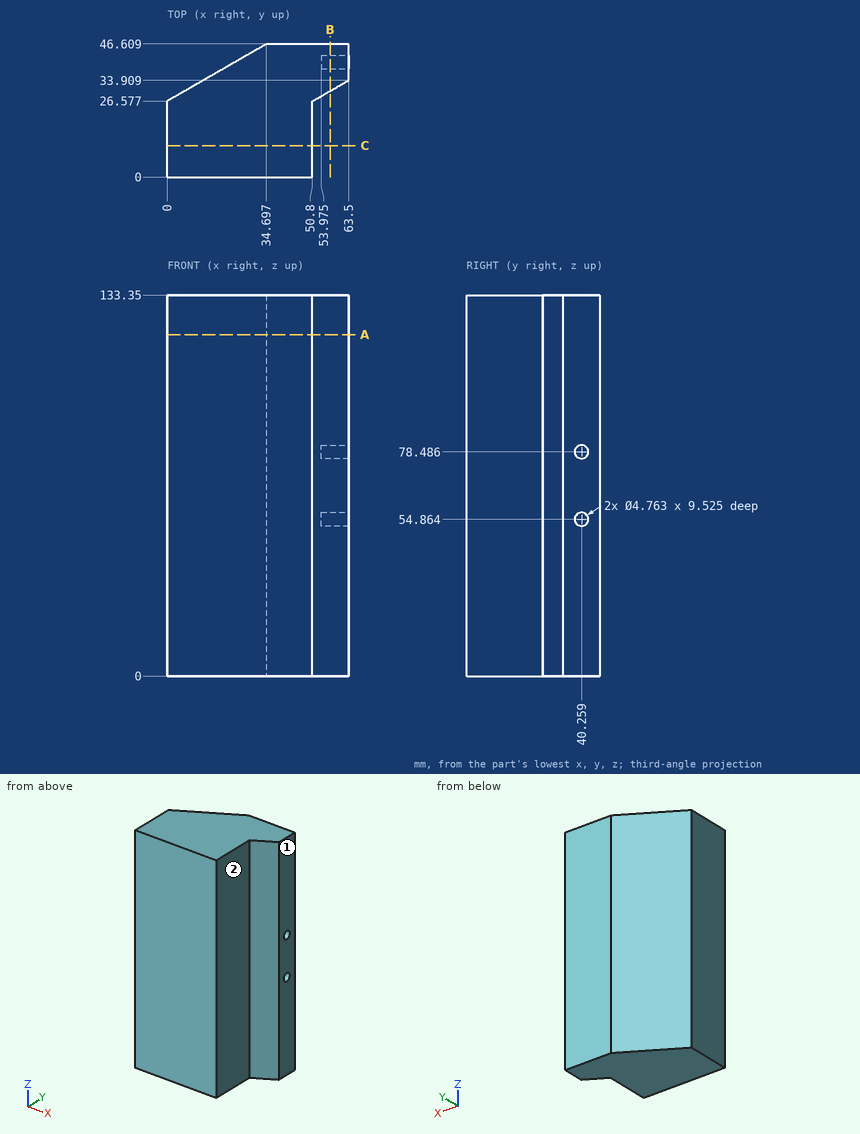
Can you work these out from the drawing? Everything is in mm from the part's minimum corner. A direction names the side the tool comes from. Round coordinates to 2 decimals unless told otherwise and drop trailing zeros. Loops run counter-clockwise (first coordinate to the right, second up) from the corner with the lowest first, then second, coordinate; pieces in that order, holes last. Notation, with made-up numbers: M 61,51 L 108,51 A10 cw 108,65 Z; hole C 3,-27.75 d8. An arc over 180 degrees is marked long. Write item = value, one per line.
1. Which directions (+Z, -Z, +X, -X, +Y, -Y) give clear straight access to the entire face, cutting with the end or side of a thin tool? Please do the marked faces 1 and 2.
Results below:
face_1 = +Z, -Z, +X, +Y, -Y
face_2 = +Z, -Z, +X, -Y
2. I need wall thicknesses on probe 1 along X at (y, z) = (12.5, 41); probe 2 along Y at (x, z) = (34, 120) (1 decimal); probe 3 along X at (y, z) = (28.5, 113.5) (1 decimal). Which ranges of each line are inside material? Lowest first, please.
Results below:
probe_1 = 0 to 50.8
probe_2 = 0 to 46.2
probe_3 = 3.3 to 54.1
3. I want a section at A-A, the plane z = 119.5. Write out the boundary of the cut face in (x, y), and give its area (3 significant figures).
Results below:
outline = M 0,0 L 50.8,0 L 50.8,26.58 L 63.5,33.91 L 63.5,46.61 L 34.7,46.61 L 0,26.58 Z
area = 2,230 mm²
4. I want a section at B-B, the plane x = 57. Count the separate pieces of the cut face and the enclosed holes in it, and give its area (3 significant figures).
Results below:
separate_pieces = 1
enclosed_holes = 2
area = 2,160 mm²
5. Will these pins go through, and if not, where does the flat tip stop? P1, Ø13.5, axis at y = 12.5, z = 64, coming from the +X side; P2, Ø4, axis at y = 40.259, z = 54.864, coming from the +X side (1 decimal); P3, Ø2, axis at y = 34, z = 60, coming from the -X side (1 decimal); P4, Ø6, axis at x = 43.5, y = 35, coming from the -Z side.
Results below:
P1 = 50.8
P2 = 54
P3 = 11.1
P4 = 0
6. I want a section at C-C, the plane y = 11. Write out the boundary of the cut face in (x, z), and give its area (3 significant figures).
Results below:
outline = M 0,0 L 50.8,0 L 50.8,133.35 L 0,133.35 Z
area = 6,770 mm²
